from build123d import *

# Parameters (mm, degrees)
BOSS_EXTRUDE1_DEPTH = 15
FILLET2_R           = 10
SHELL1_T            = -4
SKETCH7_R           = 1
BOSS_EXTRUDE4_DEPTH = 5


with BuildPart() as part:
    # Sketch1 → Boss-Extrude1 (new body)
    with BuildSketch(Plane(origin=(0, 0, 0), x_dir=(1, 0, 0), z_dir=(0, 1, 0))):
        with BuildLine():
            Line((-24, 90.710678119), (24, 90.710678119))
            ThreePointArc((24, 90.710678119), (24.707106781, 90.4177849), (25, 89.710678119))
            Line((25, 89.710678119), (25, 70.710678119))
            ThreePointArc((25, 70.710678119), (0, -75), (-25, 70.710678119))
            Line((-25, 70.710678119), (-25, 89.710678119))
            ThreePointArc((-25, 89.710678119), (-24.707106781, 90.4177849), (-24, 90.710678119))
        make_face()
    extrude(amount=BOSS_EXTRUDE1_DEPTH)

    # Fillet2
    fillet2_edges = [part.edges().sort_by_distance(p)[0] for p in [
        (25, 7.5, -70.710678119),
        (-25, 7.5, -70.710678119),
    ]]
    fillet(fillet2_edges, radius=FILLET2_R)

    # Shell1
    shell1_openings = [part.faces().sort_by_distance(p)[0] for p in [
        (0, 15, -3.849203435),
    ]]
    offset(amount=SHELL1_T, openings=shell1_openings)

    # Sketch7 → Boss-Extrude4 (add)
    with BuildSketch(Plane(origin=(0, 15, 0), x_dir=(1, 0, 0), z_dir=(0, 1, 0))):
        with Locations(Location((-73, 0, 0), (0, 0, 90))):  # turned: the seam where the file's is
            Circle(SKETCH7_R)
        with Locations(Location((73, 0, 0), (0, 0, 90))):  # turned: the seam where the file's is
            Circle(SKETCH7_R)
    extrude(amount=BOSS_EXTRUDE4_DEPTH)


solid = part.part
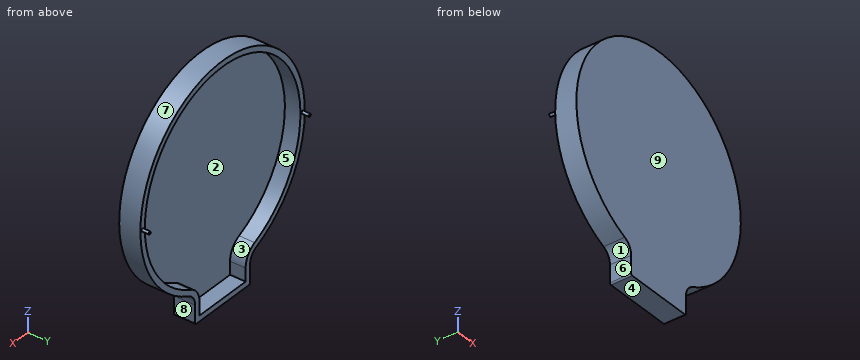
Could you check a few things on this model? Use its own coordinates, in mm. Face numbers are marked on the shaded views. A direction names the side the tool comes from. Coordinates: 2 decimals unless noted, no trailing zeros. Order: outer loops, then holes, each group sorted by start corner. A loop starts at its lowest first (then second) coordinate and runs counter-clockwise, first axis right, second up. Notation, with made-up numbers: (-9, 28) -> (23, 28) arc R21 cw to (23, 36) -> close; hole circle Ø4 at (-7, -37). An arc over 180 degrees is marked (long way). One line per item, written item: value. Start each with the question number.
1) Imagine slicing it at A-A on y = 11. List the corners of the cut face in (x, z) for me.
2) I'm going to push flat-ended pins straight in: pin 1 (6 mm diameter, centred on x = -56, z = 52, fed in from +Y); pin 2 (6 mm diameter, centred on x = -23, y = 8.5, fed in from +Z); pin 3 (3.5 mm diameter, centred on y = 6.5, z = -80.5, fed in from -X). Where does each tip first touch, or does it pass through?
3) Imagine slicing it at C-C on z = -23.5. List the corners of the cut face in (x, y) for me.
4) We'd pull the mould along X, two halves only. Please class the marked faces 1, 2, 3 and 4: +X half, -X half, draft (parallel to the pull), parting line (faces both ways), or undercut.
5) Imagine slicing it at B-B on x = 0. List the corners of the cut face in (y, z) for me, plus the area to 3 significant figures.
6) Which directions (+Z, -Z, +X, -X, +Y, -Y) give clear straight access to the entire face, cutting with the end or side of a thin tool? Please do the marked faces 5, 6, 7, 8 and 9.
7) If I drill on L1, parallel to Z at x = 0, y = 11; L2, parallel to X at y = 12.5, z = 0; L3, parallel to Y at x = 21.5, z = -77, over which ranges is the centre line in solid material (lowest first)? Write a range as [from, to].
Answer list:
1. outline: (-30.88, -68.35) arc R10 cw to (-25, -77.46) -> (-25, -89.71) arc R1 ccw to (-24, -90.71) -> (24, -90.71) arc R1 ccw to (25, -89.71) -> (25, -77.46) arc R10 cw to (30.88, -68.35) arc R75 ccw (long way) to start; hole (-29.24, -64.7) arc R14 cw to (-21, -77.46) -> (-21, -86.71) -> (21, -86.71) -> (21, -77.46) arc R14 cw to (29.24, -64.7) arc R71 ccw (long way) to start
2. pin 1: stops at y = 15
2. pin 2: stops at z = 72.28
2. pin 3: stops at x = -25
3. outline: (-71.22, 0) -> (71.22, 0) -> (71.22, 15) -> (67, 15) -> (67, 4) -> (-67, 4) -> (-67, 15) -> (-71.22, 15) -> close
4. face 1: -X half
4. face 2: undercut
4. face 3: undercut
4. face 4: draft
5. outline: (0, -90.71) -> (15, -90.71) -> (15, -86.71) -> (4, -86.71) -> (4, 71) -> (15, 71) -> (15, 75) -> (0, 75) -> close
5. area: 751 mm2
6. face 5: +Y
6. face 6: -Z, -X, +Y, -Y
6. face 7: +Y, -Y
6. face 8: -Z, +X, +Y, -Y
6. face 9: +Z, -Z, +X, -X, -Y
7. L1: z = [-90.71, -86.71], [71, 75]
7. L2: x = [-75, -71], [71, 75]
7. L3: y = [0, 15]
